```python
from build123d import *

# Parameters (mm, degrees)
F1_DEPTH  = 92
F2_T      = -2.5
F4_E13_W  = 76.4850056171
F4_E13_H  = 90
F5_DEPTH  = 10
F7_E14_W  = 15.5262811482
F7_E14_H  = 90
F8_DEPTH  = 10
F9_W      = 41.4156280458
F9_H      = 80.5949582718
F10_DEPTH = 25
F12_W     = 45.5428082496
F12_H     = 87.5177572016
F13_DEPTH = 25
F14_W     = 77.7512546629
F14_H     = 42.4544923007
F15_DEPTH = 25
F16_W     = 35.3893190622
F16_H     = 128.1821280718
F17_DEPTH = 25


with BuildPart() as f1:
    # F0 (on Top) → F1 (new body)
    with BuildSketch(Plane.XY):
        Polygon((22.0979973674, 49.8246140778), (22.0979973674, -110.3982031345), (89.0265107155, -110.3982031345), (89.0265107155, 49.8246140778), (158.6511880159, 49.8246140778), (158.6511880159, 212.2613489628), (0, 212.2613489628), (-121.0884749889, 212.2613489628), (-121.0884749889, 49.8246140778), (0, 49.8246140778), align=None)
    extrude(amount=F1_DEPTH)

    # F2
    f2_openings = [f1.faces().sort_by_distance(p)[0] for p in [
        (25.804053, 100.239761, 92),
    ]]
    offset(amount=F2_T, openings=f2_openings, kind=Kind.INTERSECTION)

    # F4_E13 (on explicit) → F5 (join)
    with BuildSketch(Plane(origin=(4.0378416888, 209.7613489628, 2.5), x_dir=(0, -1, 0), z_dir=(-1, 0, 0))):
        with Locations((38.2425028086, 45)):
            Rectangle(F4_E13_W, F4_E13_H)
    extrude(amount=F5_DEPTH)

    # F7_E14 (on explicit) → F8 (join)
    with BuildSketch(Plane(origin=(0, 52.3246140778, 2.5), x_dir=(0, 1, 0), z_dir=(1, 0, 0))):
        with Locations((7.7631405741, 45)):
            Rectangle(F7_E14_W, F7_E14_H)
    extrude(amount=F8_DEPTH)

    # F9 (on face) → F10 (cut)
    with BuildSketch(Plane.XZ.offset(110.3982031345)):
        with Locations((53.3959884197, 44.4829904009)):
            Rectangle(F9_W, F9_H)
    extrude(amount=-F10_DEPTH, mode=Mode.SUBTRACT)

    # F12 (on face) → F13 (cut)
    with BuildSketch(Plane(origin=(0, 212.2613489628, 0), x_dir=(-1, 0, 0), z_dir=(0, 1, 0))):
        with Locations((-41.2379493937, 45.8978245733)):
            Rectangle(F12_W, F12_H)
    extrude(amount=-F13_DEPTH, mode=Mode.SUBTRACT)

    # F14 (on face) → F15 (cut)
    with BuildSketch(Plane.XZ.offset(-209.7613489628)):
        with Locations((-60.8778791502, 59.6545059234)):
            Rectangle(F14_W, F14_H)
    extrude(amount=-F15_DEPTH, mode=Mode.SUBTRACT)

    # F16 (on face) → F17 (join)
    with BuildSketch(Plane.XY.offset(2.5)):
        Polygon((155.4546654224, 209.2887163162), (71.6699585319, 209.2887163162), (71.6699585319, 181.543186307), (120.0653463602, 181.543186307), (155.4546654224, 181.543186307), align=None)
        with Locations((137.7600058913, 117.4521222711)):
            Rectangle(F16_W, F16_H)
    extrude(amount=F17_DEPTH)


solid = f1.part
```
Design review of the part built by this model. Coordinates are the model's own, in mm. A direction names the side the tool comes from. Coordinates: 2 decimals unless noted, no trailing zeros. Loops run counter-clockwise (first coordinate to the right, second up) from the corner with the lowest first, then second, coordinate; pieces in that order, holes last. Notation, with made-up numbers: M 74.25,23.5 L 125.25,23.5 A34 ccw 125.25,53.5 Z; hole C 15.5,10 d3. An arc over 180 degrees is marked long. One line per question, with ' | ' between items.
(1) We need section B-B (y = -73). Give the boundary of the cut face in (x, z).
Filled in:
outline: M 22.1,0 L 89.03,0 L 89.03,92 L 86.53,92 L 86.53,2.5 L 24.6,2.5 L 24.6,92 L 22.1,92 Z
(2) Draft analysis for pull direction X (two halves, no side actions). For faces 1 (the face through (76, -107.898, 57)), 2 (the face through (158.651, 130, 45)), 3 (the face through (-10, 212.261, 45)), state which applies: released by +X, released by -X, zero draft, split by the parting line, or undercut.
Filled in:
face 1: undercut | face 2: released by +X | face 3: zero draft
(3) Wall thickness on probe 1 along Y at (x, z) = (139.5, 20); probe 2 along Y at (x, z) = (91.5, 26); probe 3 along X at (y, z) = (149.5, 44): over which ranges is each line inside the solid? List them lowest first.
Filled in:
probe 1: y = 49.82 to 52.32, 53.36 to 209.29, 209.76 to 212.26 | probe 2: y = 49.82 to 52.32, 181.54 to 209.29, 209.76 to 212.26 | probe 3: x = -121.09 to -118.59, -5.96 to 4.04, 156.15 to 158.65
(4) We need section C-C (z = 9). Count the separate pieces of the cut face and the enclosed holes in it, and give its area (3 significant figures).
Filled in:
separate pieces: 3 | enclosed holes: 0 | area: 10,600 mm^2
(5) Machinability: for faces 4 (the face through (155.455, 130, 15)), 5 (the face through (-1, 172, 92.5)), 6 (the face through (77, -110.398, 56)), 7 (the face through (89.027, -31, 45)), 8 (the face through (18.467, 211, 46)), which of the approach directions +Z, -Z, +X, -X, +Y, -Y give a long, thin tool a straight path to every point of the face, cutting with its end or side? Answer none if there is none.
Filled in:
face 4: +Z | face 5: +Z, +X, -X, +Y, -Y | face 6: +Z, -Z, +X, -X, -Y | face 7: +Z, -Z, +X, -Y | face 8: +Y
(6) We need section D-D (y = 109). Give the boundary of the cut face in (x, z).
Filled in:
outline: M -121.09,0 L 158.65,0 L 158.65,92 L 156.15,92 L 156.15,2.5 L 155.45,2.5 L 155.45,27.5 L 120.07,27.5 L 120.07,2.5 L -118.59,2.5 L -118.59,92 L -121.09,92 Z
(7) We need section A-A (x = 51). Give the boundary of the cut face in (y, z), and give its area (3 significant figures).
Filled in:
outline: M -110.4,0 L 212.26,0 L 212.26,2.14 L 187.26,2.14 L 187.26,2.5 L -107.9,2.5 L -107.9,4.19 L -110.4,4.19 Z; M -110.4,84.78 L -107.9,84.78 L -107.9,92 L -110.4,92 Z; M 209.76,89.66 L 212.26,89.66 L 212.26,92 L 209.76,92 Z | area: 826 mm^2
(8) For pin 1 Ø2 at (y, z) = (40, 68.5) entering from -X; pin 2 Ø1.5 at (x, y) = (120.5, 172.5) entering from +Z; pin 3 Ø3 at (y, z) = (-109, 40.5) entering from +X, all flat-tipped, find the tip position at first contact; note any pin that passes through.
Filled in:
pin 1: stops at x = 22.1 | pin 2: stops at z = 27.5 | pin 3: stops at x = 89.03
